For this review, use the dimensioned drawing (mm, ordinates from the lowest corner) and the shaded views. Coordinates: 2 decimals unless noted, no trailing zeros. Loops run counter-clockwise (first coordinate to the right, second up) from the corner with the lowest first, then second, coordinate; pieces in that order, holes last. Notation, with made-up numbers: (-11, -6.75) - (39, -6.75) arc R20 cw to (39, 30.25) - close; hole circle Ø9 at (-26.5, -9.75). An arc over 180 degrees is marked (long way). One line per item, written item: value. Start each with the question number.
1. We need section B-B, the plane x = 75. Give the boundary of the cut face in (y, z) (3 decimals), then the cut area to 3 significant figures.
2. We need section D-D, the plane y = 26. Give the boundary of the cut face in (x, z) (3 decimals).
3. To check wall thickness, follow line 1 (X direction, y = 17.5, z = 0.35); line 2 (X direction, y = 20.5, z = 1.1); line 3 (X direction, y = 10.5, z = 0.35). State the ranges of each line that lie inside material, in increasing order.
4. We need section C-C, the plane z = 2.4. Give the boundary of the cut face in (x, y) (3 decimals).
5. We need section A-A, the plane y = 20. Give the boundary of the cut face in (x, z) (3 decimals), then the cut area to 3 significant figures.
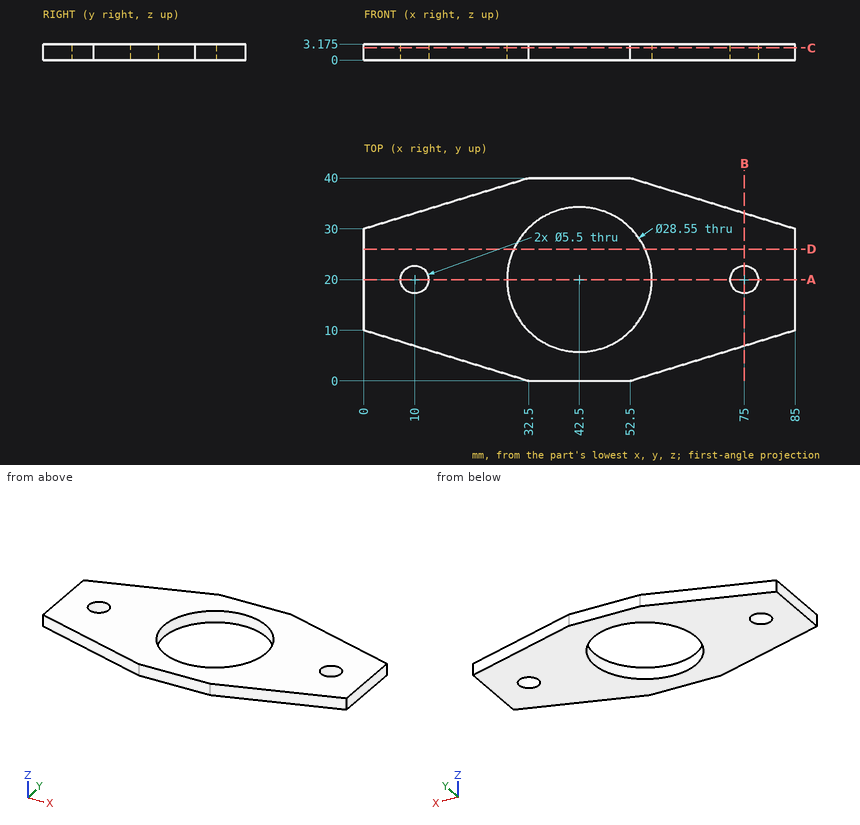
Findings below:
1. outline: (6.923, 0) - (17.25, 0) - (17.25, 3.175) - (6.923, 3.175) - close; (22.75, 0) - (33.077, 0) - (33.077, 3.175) - (22.75, 3.175) - close
1. area: 65.6 mm2
2. outline: (0, 0) - (29.547, 0) - (29.547, 3.175) - (0, 3.175) - close; (55.453, 0) - (85, 0) - (85, 3.175) - (55.453, 3.175) - close
3. line 1: 0 to 8.85, 11.15 to 28.45, 56.55 to 73.85, 76.15 to 85
3. line 2: 0 to 7.3, 12.7 to 28.23, 56.77 to 72.3, 77.7 to 85
3. line 3: 0 to 31.85, 53.15 to 85
4. outline: (0, 10) - (32.5, 0) - (52.5, 0) - (85, 10) - (85, 30) - (52.5, 40) - (32.5, 40) - (0, 30) - close; hole circle Ø5.5 at (10, 20); hole circle Ø28.55 at (42.5, 20); hole circle Ø5.5 at (75, 20)
5. outline: (0, 0) - (7.25, 0) - (7.25, 3.175) - (0, 3.175) - close; (12.75, 0) - (28.225, 0) - (28.225, 3.175) - (12.75, 3.175) - close; (56.775, 0) - (72.25, 0) - (72.25, 3.175) - (56.775, 3.175) - close; (77.75, 0) - (85, 0) - (85, 3.175) - (77.75, 3.175) - close
5. area: 144 mm2
